```python
from build123d import *

# Parameters (mm, degrees)
OUTPUT_MASTER_SKETCH_R   = 25.05
BOSS_EXTRUDE1_DEPTH      = 9
SKETCH4_R                = 2.85
CUT_EXTRUDE1_DEPTH       = 4
SKETCH5_R                = 25.55
SKETCH5_R_2              = 25.05
BOSS_EXTRUDE2_DEPTH      = 0.5
SKETCH6_R                = 1.55
CUT_EXTRUDE2_DEPTH       = 38.237145433
CUT_EXTRUDE3_START       = -3.1
SKETCH7_R                = 2.85
CUT_EXTRUDE3_DEPTH       = 3.1
CHAMFER1_SIZE            = 0.5
SKETCH10_R               = 2.1
M4_THRU_DEPTH            = 38.237145433
CUT_EXTRUDE4_DEPTH       = 5
FILLET1_R                = 1
CIRPATTERN1_COUNT        = 6
FILLET1_OF_CIRPATTERN1_R = 1


with BuildPart() as part:
    # Output Master Sketch → Boss-Extrude1 (new body)
    with BuildSketch(Plane.XY):
        Circle(OUTPUT_MASTER_SKETCH_R)
    extrude(amount=BOSS_EXTRUDE1_DEPTH)

    # Sketch4 → Cut-Extrude1 (cut)
    with BuildSketch(Plane.XY):
        with Locations((21, 0)):
            Circle(SKETCH4_R)
        with Locations((10.5, -18.186533479)):
            Circle(SKETCH4_R)
        with Locations((-10.5, -18.186533479)):
            Circle(SKETCH4_R)
        with Locations((-21, 0)):
            Circle(SKETCH4_R)
        with Locations((-10.5, 18.186533479)):
            Circle(SKETCH4_R)
        with Locations((10.5, 18.186533479)):
            Circle(SKETCH4_R)
    extrude(amount=CUT_EXTRUDE1_DEPTH, mode=Mode.SUBTRACT)

    # Sketch5 → Boss-Extrude2 (add)
    with BuildSketch(Plane(origin=(0, 0, 0), x_dir=(-1, 0, 0), z_dir=(0, 0, -1))):
        Circle(SKETCH5_R)
        Circle(SKETCH5_R_2, mode=Mode.SUBTRACT)
    extrude(amount=-BOSS_EXTRUDE2_DEPTH)

    # Sketch6 → Cut-Extrude2 (cut, through all)
    with BuildSketch(Plane(origin=(0, 0, 0), x_dir=(-1, 0, 0), z_dir=(0, 0, -1))):
        with Locations((-21, 0)):
            Circle(SKETCH6_R)
        with Locations((-10.5, 18.186533479)):
            Circle(SKETCH6_R)
        with Locations((10.5, 18.186533479)):
            Circle(SKETCH6_R)
        with Locations((21, 0)):
            Circle(SKETCH6_R)
        with Locations((10.5, -18.186533479)):
            Circle(SKETCH6_R)
        with Locations((-10.5, -18.186533479)):
            Circle(SKETCH6_R)
    extrude(amount=-CUT_EXTRUDE2_DEPTH, mode=Mode.SUBTRACT)

    # Sketch7 → Cut-Extrude3 (cut)
    with BuildSketch(Plane.XY.offset(9).offset(CUT_EXTRUDE3_START)):
        with Locations((-21, 0)):
            Circle(SKETCH7_R)
        with Locations((-10.5, 18.186533479)):
            Circle(SKETCH7_R)
        with Locations((10.5, 18.186533479)):
            Circle(SKETCH7_R)
        with Locations((21, 0)):
            Circle(SKETCH7_R)
        with Locations((10.5, -18.186533479)):
            Circle(SKETCH7_R)
        with Locations((-10.5, -18.186533479)):
            Circle(SKETCH7_R)
    extrude(amount=CUT_EXTRUDE3_DEPTH, mode=Mode.SUBTRACT)

    # Chamfer1
    chamfer1_edges = [part.edges().sort_by_distance(p)[0] for p in [
        (-25.05, 0, 9),
    ]]
    chamfer(chamfer1_edges, length=CHAMFER1_SIZE)

    # Sketch10 → M4 Thru (cut, through all)
    with BuildSketch(Plane.XY.offset(9)):
        with Locations((0, 20)):
            Circle(SKETCH10_R)
        with Locations((17.320508076, 10)):
            Circle(SKETCH10_R)
        with Locations((17.320508076, -10)):
            Circle(SKETCH10_R)
        with Locations((0, -20)):
            Circle(SKETCH10_R)
        with Locations((-17.320508076, -10)):
            Circle(SKETCH10_R)
        with Locations((-17.320508076, 10)):
            Circle(SKETCH10_R)
    extrude(amount=-M4_THRU_DEPTH, mode=Mode.SUBTRACT)

    # Sketch12 → Cut-Extrude4 (cut)
    with BuildSketch(Plane.XY.offset(9)):
        with BuildLine():
            Line((0, 7.5), (0, 15))
            ThreePointArc((0, 15), (-2.92635483, 14.711779206), (-5.740251485, 13.858192988))
            Line((-5.740251485, 13.858192988), (-2.870125743, 6.929096494))
            ThreePointArc((-2.870125743, 6.929096494), (-1.463177415, 7.355889603), (0, 7.5))
        make_face()
        with BuildLine():
            ThreePointArc((5.740251485, 13.858192988), (2.92635483, 14.711779206), (0, 15))
            Line((0, 15), (0, 7.5))
            ThreePointArc((0, 7.5), (1.463177415, 7.355889603), (2.870125743, 6.929096494))
            Line((2.870125743, 6.929096494), (5.740251485, 13.858192988))
        make_face()
    cut_extrude4 = extrude(amount=-CUT_EXTRUDE4_DEPTH, mode=Mode.SUBTRACT)

    # Fillet1
    fillet1_edges = [part.edges().sort_by_distance(p)[0] for p in [
        (2.870125743, 6.929096494, 6.5),
        (-2.870125743, 6.929096494, 6.5),
        (-5.740251485, 13.858192988, 6.5),
        (5.740251485, 13.858192988, 6.5),
    ]]
    fillet(fillet1_edges, radius=FILLET1_R)

    # CirPattern1: Cut-Extrude4 ×6 about axis
    cirpattern1_axis = Axis((0, 0, 0), (0, 0, 1))
    for i in range(1, CIRPATTERN1_COUNT):
        add(cut_extrude4.rotate(cirpattern1_axis, i * 360 / CIRPATTERN1_COUNT), mode=Mode.SUBTRACT)

    # Fillet1 of CirPattern1
    fillet1_of_cirpattern1_edges = [part.edges().sort_by_distance(p)[0] for p in [
        (-4.565710718, 5.950150052, 6.5),
        (-7.43583646, 0.978946442, 6.5),
        (-14.871672921, 1.957892883, 6.5),
        (-9.131421435, 11.900300104, 6.5),
        (-7.43583646, -0.978946442, 6.5),
        (-4.565710718, -5.950150052, 6.5),
        (-9.131421435, -11.900300104, 6.5),
        (-14.871672921, -1.957892883, 6.5),
        (-2.870125743, -6.929096494, 6.5),
        (2.870125743, -6.929096494, 6.5),
        (5.740251485, -13.858192988, 6.5),
        (-5.740251485, -13.858192988, 6.5),
        (4.565710718, -5.950150052, 6.5),
        (7.43583646, -0.978946442, 6.5),
        (14.871672921, -1.957892883, 6.5),
        (9.131421435, -11.900300104, 6.5),
        (7.43583646, 0.978946442, 6.5),
        (4.565710718, 5.950150052, 6.5),
        (9.131421435, 11.900300104, 6.5),
        (14.871672921, 1.957892883, 6.5),
    ]]
    fillet(fillet1_of_cirpattern1_edges, radius=FILLET1_OF_CIRPATTERN1_R)


solid = part.part
```
Here's how the part is built. I have some questions about the finished solid (model axes, mm). A direction names the side the tool comes from. Coordinates: 2 decimals unless noted, no trailing zeros. Return JSON: item names as keys, results as strings. Group by question number.
Item 1: On a 3-axis mill with a long thin cutter (end or side, diameter ignored), from which of +Z, -Z, +X, -X, +Y, -Y can I reach the whole of each face in a straight line? I mean faces 1 (the face through (-9, -19, 4)), 2 (the face through (-15.317, 10.631, 4.563)), 3 (the face through (-10, 6, 4)). Say none if no direction works.
Item 2: I need wall thicknesses on line 1 (X direction, y = 2, z = 8); line 2 (Y direction, x = -17.5, z = 2.5); line 3 (X direction, y = 9, z = 5.25). Which ranges of each line are inside material? Lowest first, please. Write a range as from..to.
Item 3: If we section it at A-A on y = 0: State how many separate pieces and enclosed holes the cut face has, and give its area (3 significant figures).
Item 4: Will these pins go through, and if not, where does the flat tip stop? P1, Ø3.5, axis at x = -10.5, y = -18.19, coming from the +Z side; P2, Ø5, axis at x = 10.5, y = 18.19, coming from the -Z side; P3, Ø4, axis at x = -7.5, z = 2, coming from the -Y side.
Calculated:
{
 "1": {"face 1": "-Z", "face 2": "+Z, -Z", "face 3": "+Z"},
 "2": {"line 1": "x = -24.97..-23.03, -18.97..-14.29, -7.23..7.23, 14.29..18.97, 23.03..24.97", "line 2": "y = -17.92..-12.09, -7.91..7.91, 12.09..17.92", "line 3": "x = -23.38..-19.17, -15.47..-12, -6.91..-3.73, 3.73..6.91, 12..15.47, 19.17..23.38"},
 "3": {"separate pieces": "3", "enclosed holes": "0", "area": "358 mm^2"},
 "4": {"P1": "stops at z = 5.9", "P2": "stops at z = 4", "P3": "stops at y = -24.79"}
}
